```python
from build123d import *

# Parameters (mm, degrees)
BOSS_EXTRUDE1_DEPTH = 3.175
CUT_EXTRUDE4_DEPTH  = 235.179100055
FILLET1_R           = 25.4
BOSS_EXTRUDE2_DEPTH = 3.175


with BuildPart() as part:
    # Sketch1 → Boss-Extrude1 (new body)
    with BuildSketch(Plane(origin=(0, 0, 0), x_dir=(1, 0, 0), z_dir=(0, 1, 0))):
        Polygon((-139.7, 73.520142619), (-121.739487758, 91.480654861), (121.739487758, 91.480654861), (139.7, 73.520142619), (139.7, -169.958832897), (121.739487758, -187.919345139), (-121.739487758, -187.919345139), (-139.7, -169.958832897), align=None)
    extrude(amount=BOSS_EXTRUDE1_DEPTH)

    # Sketch2 → Cut-Extrude4 (cut, through all)
    with BuildSketch(Plane(origin=(0, 3.175, 0), x_dir=(1, 0, 0), z_dir=(0, 1, 0))):
        Polygon((-103.778975516, 37.599118134), (-114.3, 27.07809365), (-114.3, -123.516783928), (-103.778975516, -134.037808413), (-85.818463274, -151.998320655), (-75.297438789, -162.519345139), (75.297438789, -162.519345139), (85.818463274, -151.998320655), (103.778975516, -134.037808413), (114.3, -123.516783928), (114.3, 27.07809365), (103.778975516, 37.599118134), (85.818463274, 55.559630377), (75.297438789, 66.080654861), (-75.297438789, 66.080654861), (-85.818463274, 55.559630377), align=None)
    extrude(amount=-CUT_EXTRUDE4_DEPTH, mode=Mode.SUBTRACT)

    # Fillet1
    fillet1_edges = [part.edges().sort_by_distance(p)[0] for p in [
        (-75.297438789, 1.5875, -66.080654861),
        (75.297438789, 1.5875, -66.080654861),
        (114.3, 1.5875, -27.07809365),
        (114.3, 1.5875, 123.516783928),
        (75.297438789, 1.5875, 162.519345139),
        (-75.297438789, 1.5875, 162.519345139),
        (-114.3, 1.5875, 123.516783928),
        (-114.3, 1.5875, -27.07809365),
    ]]
    fillet(fillet1_edges, radius=FILLET1_R)

    # Sketch6 → Boss-Extrude2 (add)
    with BuildSketch(Plane(origin=(0, 3.175, 0), x_dir=(1, 0, 0), z_dir=(0, 1, 0))):
        Polygon((50.8, 2.580654861), (139.7, 2.580654861), (139.7, -111.719345139), (-139.7, -111.719345139), (-139.7, 2.580654861), (-139.7, 73.520142619), (50.8, 73.520142619), align=None)
    extrude(amount=-BOSS_EXTRUDE2_DEPTH)


solid = part.part
```
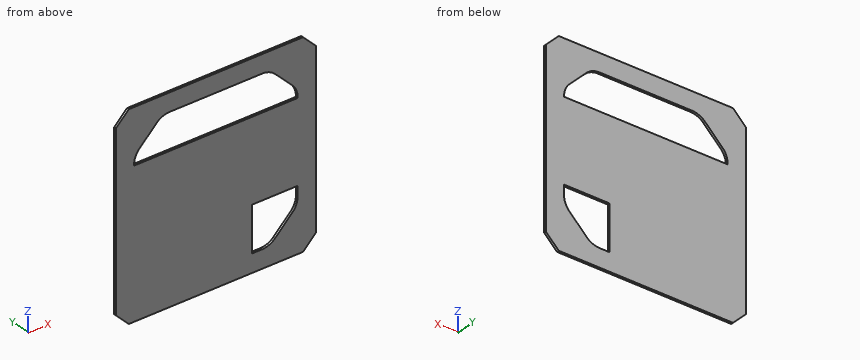
The listing builds one solid part. Answer for the finished solid, in the listing's coordinates (mm). Coordinates: 2 decimals unless noted, no trailing zeros. Write each loop counter-clockwise with the first axis right and the second up, starting at its lowest first coordinate (ties: lowest second). Pieces come first, ordered by that corner, then holes.
Q1. Section A-A, the plane x = -54 is taken. Write down the section's boundary in (y, z) (3 decimals).
Returned:
outline: (0, -91.481) - (3.175, -91.481) - (3.175, 111.719) - (0, 111.719) - close; (0, 162.519) - (3.175, 162.519) - (3.175, 187.919) - (0, 187.919) - close
Q2. Section C-C, the plane z = 120.5 is taken. Write down the section's boundary in (x, y) (3 decimals).
Returned:
outline: (-139.7, 0) - (-113.166, 0) - (-113.166, 3.175) - (-139.7, 3.175) - close; (113.166, 0) - (139.7, 0) - (139.7, 3.175) - (113.166, 3.175) - close
Q3. Section D-D, the plane x = 94 is taken. Write down the section's boundary in (y, z) (3 decimals).
Returned:
outline: (0, -91.481) - (3.175, -91.481) - (3.175, -47.378) - (0, -47.378) - close; (0, -2.581) - (3.175, -2.581) - (3.175, 111.719) - (0, 111.719) - close; (0, 143.817) - (3.175, 143.817) - (3.175, 187.919) - (0, 187.919) - close
Q4. Find the intervals of material crossed by line 1 along Z through (x, y) = (53, 1.3); line 2 along Z through (x, y) = (-62.5, 0.2); line 3 along Z through (x, y) = (74, 0.85), in increasing order.
Returned:
line 1: z = -91.48 to -66.08, -2.58 to 111.72, 162.52 to 187.92
line 2: z = -91.48 to 111.72, 162.52 to 187.92
line 3: z = -91.48 to -64.35, -2.58 to 111.72, 160.79 to 187.92
Q5. Section B-B, the plane y = 0.65 is taken. Write down the section's boundary in (x, z).
Returned:
outline: (-139.7, -73.52) - (-121.74, -91.48) - (121.74, -91.48) - (139.7, -73.52) - (139.7, 169.96) - (121.74, 187.92) - (-121.74, 187.92) - (-139.7, 169.96) - close; hole (-114.3, 111.72) - (114.3, 111.72) - (114.3, 113) arc R25.4 ccw to (106.86, 130.96) - (82.74, 155.08) arc R25.4 ccw to (64.78, 162.52) - (-64.78, 162.52) arc R25.4 ccw to (-82.74, 155.08) - (-106.86, 130.96) arc R25.4 ccw to (-114.3, 113) - close; hole (50.8, -66.08) - (64.78, -66.08) arc R25.4 ccw to (82.74, -58.64) - (106.86, -34.52) arc R25.4 ccw to (114.3, -16.56) - (114.3, -2.58) - (50.8, -2.58) - close
